For this review, take the finished solid that the model builds, in its own axes (mm). A direction names the side the tool comes from. Coordinates: 2 decimals unless noted, no trailing zeros. Loops run counter-clockwise (first coordinate to the right, second up) from the corner with the lowest first, then second, coordinate; pieces in that order, holes last.
1. Take a section at C-C, the plane z = 43. State the section outline as (x, y) points, then the cut area to 3 significant figures.
2. To check wall thickness, follow probe 1 along X at (y, z) = (1.35, 27); probe 2 along X at (y, z) = (1.7, -8); probe 3 along X at (y, z) = (1.75, 43). State the ranges of each line that lie inside material, in increasing order.
3. Mouldability with a two-part tool opening along X and no side actions: class faces 1 (the face through (0.07, 1.48, 3.25)), 2 (the face through (-36, 1, -26.5)), 3 (the face through (6.9, 1.52, -25.93)) as pulls with the +X half, pulls with the -X half, needs draft (parallel to the pull), parting line crosses it, or undercut.
4. Machinability: for faces 4 (the face through (3.25, 1, -5)), 5 (the face through (7.5, 1, 13)), which of the approach directions +Z, -Z, +X, -X, +Y, -Y give a long, thin tool a straight path to every point of the face, cutting with its end or side? Answer none if there is none.
5. Take a section at B-B, the plane y = 0.8. State the section outline as (x, z) points.
6. Take a section at D-D, the plane z = -19. State the section outline as (x, y) points, then the cut area to 3 significant figures.
7. Clearance check with flat-ended pins moving along their axes: P1, Ø1.5, axis at y = 1.5, z = 7, coming from the -X side; P2, Ø3, axis at x = 0, z = -18.5, coming from the +Y side. State where each tip first meets the part, or that it passes through.
8. Take a section at A-A, the plane x = 0. State the section outline as (y, z) points.
```python
from build123d import *

# Parameters (mm, degrees)
SKETCH_1_R      = 1.65
SKETCH_1_R_2    = 1.7
EXTRUDE_1_DEPTH = 3
FILLET_1_R      = 2


with BuildPart() as part:
    # 草图1 → 凸台-拉伸1 (new body)
    with BuildSketch(Plane(origin=(0, 0, 0), x_dir=(1, 0, 0), z_dir=(0, 1, 0))):
        Polygon((-80, 11.5), (-7.5, -52), (7.5, -52), (7.5, 26.5), (-7.5, 26.5), (-80, 26.5), align=None)
        with Locations(Location((0, 18.5, 0), (0, 0, 270))):
            Circle(SKETCH_1_R, mode=Mode.SUBTRACT)
        with Locations(Location((0, -28, 0), (0, 0, 270))):
            Circle(SKETCH_1_R, mode=Mode.SUBTRACT)
        with Locations(Location((0, -43, 0), (0, 0, 270))):
            Circle(SKETCH_1_R, mode=Mode.SUBTRACT)
        with Locations(Location((-70, 19, 0), (0, 0, 270))):
            Circle(SKETCH_1_R_2, mode=Mode.SUBTRACT)
        with Locations(Location((-50, 19, 0), (0, 0, 270))):
            Circle(SKETCH_1_R_2, mode=Mode.SUBTRACT)
        with BuildLine():
            Line((-3.25, 0), (-3.25, 10.5))
            ThreePointArc((-3.25, 10.5), (0, 13.75), (3.25, 10.5))
            Line((3.25, 10.5), (3.25, 0))
            ThreePointArc((3.25, 0), (0, -3.25), (-3.25, 0))
        make_face(mode=Mode.SUBTRACT)
        with BuildLine():
            Line((-7.5, -32.544518989), (-7.5, 7.5))
            ThreePointArc((-7.5, 7.5), (-8.671572875, 10.328427125), (-11.5, 11.5))
            Line((-11.5, 11.5), (-57.220120105, 11.5))
            ThreePointArc((-57.220120105, 11.5), (-60.964187654, 8.907820368), (-59.855607382, 4.490979094))
            Line((-59.855607382, 4.490979094), (-14.135487277, -35.553539895))
            ThreePointArc((-14.135487277, -35.553539895), (-9.848023775, -36.18745387), (-7.5, -32.544518989))
        make_face(mode=Mode.SUBTRACT)
    extrude(amount=EXTRUDE_1_DEPTH)

    # 圆角1
    fillet_1_edges = [part.edges().sort_by_distance(p)[0] for p in [
        (7.5, 1.5, 52),
        (-7.5, 1.5, 52),
        (-80, 1.5, -11.5),
        (-80, 1.5, -26.5),
        (7.5, 1.5, -26.5),
    ]]
    fillet(fillet_1_edges, radius=FILLET_1_R)


solid = part.part
```
Results list:
1. outline: (-17.78, 0) - (-1.65, 0) - (-1.65, 3) - (-17.78, 3) - close; (1.65, 0) - (7.5, 0) - (7.5, 3) - (1.65, 3) - close
1. area: 65.9 mm2
2. probe 1: x = -36.04 to -23.9, -7.5 to -1.31, 1.31 to 7.5
2. probe 2: x = -76 to -61.19, -7.53 to -3.25, 3.25 to 7.5
2. probe 3: x = -17.78 to -1.65, 1.65 to 7.5
3. face 1: undercut
3. face 2: needs draft
3. face 3: pulls with the +X half
4. face 4: +Y, -Y
4. face 5: +Z, -Z, +X, +Y, -Y
5. outline: (-80, -24.5) arc R2 ccw to (-78, -26.5) - (5.5, -26.5) arc R2 ccw to (7.5, -24.5) - (7.5, 50) arc R2 ccw to (5.5, 52) - (-6.75, 52) arc R2 ccw to (-8.07, 51.5) - (-79.32, -10.9) arc R2 ccw to (-80, -12.41) - close; hole circle Ø3.4 at (-70, -19); hole (-59.86, -4.49) arc R4 ccw to (-57.22, -11.5) - (-11.5, -11.5) arc R4 ccw to (-7.5, -7.5) - (-7.5, 32.54) arc R4 ccw to (-14.14, 35.55) - close; hole circle Ø3.4 at (-50, -19); hole (-3.25, -10.5) arc R3.25 ccw to (3.25, -10.5) - (3.25, 0) arc R3.25 ccw to (-3.25, 0) - close; hole circle Ø3.3 at (0, -18.5); hole circle Ø3.3 at (0, 28); hole circle Ø3.3 at (0, 43)
6. outline: (-80, 0) - (-71.7, 0) - (-71.7, 3) - (-80, 3) - close; (-68.3, 0) - (-51.7, 0) - (-51.7, 3) - (-68.3, 3) - close; (-48.3, 0) - (-1.57, 0) - (-1.57, 3) - (-48.3, 3) - close; (1.57, 0) - (7.5, 0) - (7.5, 3) - (1.57, 3) - close
6. area: 233 mm2
7. P1: stops at x = -59.73
7. P2: passes through
8. outline: (0, -26.5) - (3, -26.5) - (3, -20.15) - (0, -20.15) - close; (0, -16.85) - (3, -16.85) - (3, -13.75) - (0, -13.75) - close; (0, 3.25) - (3, 3.25) - (3, 26.35) - (0, 26.35) - close; (0, 29.65) - (3, 29.65) - (3, 41.35) - (0, 41.35) - close; (0, 44.65) - (3, 44.65) - (3, 52) - (0, 52) - close
